Here's how the part is built. I have some questions about the finished solid (model axes, mm). Give positions to 0.01 mm unless a question says otherwise; leave off trailing zeros. Order: outer loops, then holes, each group sorted by start corner. A loop starts at its lowest first (then second) coordinate and runs counter-clockwise, first axis right, second up.
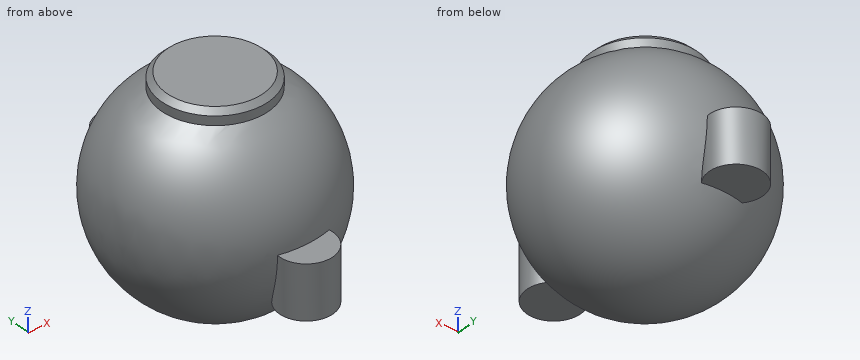
Autodesk Inventor part; units mm, degrees
sketch "スケッチ1" plane through (0, 0, 0) normal (0, 0, 1) x (1, 0, 0)
  arc A0 (0, 100) -> (0, -100) centre (0, 0) ccw
  line L0 (0, 100) -> (0, -100)
  dimension "d0" = 200
revolve "回転1" add sketch "スケッチ1" angle 360 about axis through (0, 100, 0) along (0, -1, 0)
ref_plane "作業平面1" through (0, 0, 200) normal (0, 0, 1) x (1, 0, 0)
ref_plane "作業平面2" through (0, 100, 0) normal (0, 1, 0) x (-1, 0, 0)
ref_plane "作業平面3" through (0, -100, 0) normal (0, 1, 0) x (-1, 0, 0)
ref_plane "作業平面4" through (0, 0, -100) normal (0, 0, 1) x (1, 0, 0)
sketch "スケッチ2" plane through (0, 0, 0) normal (0, 0, 1) x (1, 0, 0)
  circle A0 centre (0, 0) radius 50
  dimension "d6" = 100
extrude "押し出し1" add sketch "スケッチ2" along normal blind 100
chamfer "面取り1" distance 5 angle 45 1 edges at (-50, 0, 100)
sketch "スケッチ3" plane through (0, 0, 0) normal (0, 0, 1) x (1, 0, 0)
  circle A0 centre (0, 100) radius 25
  point P0 (0, 0)
  dimension "d12" = 50
  dimension "d13" = 100
extrude "押し出し2" add sketch "スケッチ3" against normal blind 50
mirror "ミラー1" about plane through (0, 0, 0) normal (0, 1, 0) of "押し出し2"
properties part number "Hips"
Q1. I'm going to push flat-ended pins straight in: P1, Ø8, axis at x = 47.5, y = 52.5, coming from the +Z side; P2, Ø5, axis at y = 18, z = -2, coming from the -X side; P3, Ø3, axis at y = -54.5, z = -8, coming from the +X side. Where does each tip first touch, or does it pass through?
Filled sheet:
P1: stops at z = 74.42
P2: stops at x = -98.77
P3: stops at x = 84.43
Q2. If we section it at A-A on y = 0: List the corners of the cut face in (x, z) for me, plus the area to 3 significant figures.
Filled sheet:
outline: (-50, 86.6) arc R100 ccw (long way) to (50, 86.6) - (50, 95) - (45, 100) - (-45, 100) - (-50, 95) - close
area: 31,800 mm2
Q3. If we section it at C-C on y = -109: List the corners of the cut face in (x, z) for me, plus the area to 3 significant figures.
Filled sheet:
outline: (-23.32, -50) - (23.32, -50) - (23.32, 0) - (-23.32, 0) - close
area: 2,330 mm2
Q4. If we section it at D-D on x = -75.5: List the corners of the cut face in (y, z) for me, plus the area to 3 significant figures.
Filled sheet:
outline: circle Ø131.14 at (0, 0)
area: 13,500 mm2
Q5. I need wall thicknesses on L1, parallel to Z at x = 18.5, y = -112.5; L2, parallel to X at y = 23, z = -48.5; L3, parallel to Z at x = -20, y = 2.5. Which ranges of each line are inside material? Lowest first, please.
Filled sheet:
L1: z = -50 to 0
L2: x = -84.37 to 84.37
L3: z = -97.95 to 100
Q6. If we section it at B-B on x = 0: List the corners of the cut face in (y, z) for me.
Filled sheet:
outline: (-125, -50) - (-86.6, -50) arc R100 ccw to (86.6, -50) - (125, -50) - (125, 0) - (100, 0) arc R100 ccw to (50, 86.6) - (50, 95) - (45, 100) - (-45, 100) - (-50, 95) - (-50, 86.6) arc R100 ccw to (-100, 0) - (-125, 0) - close
